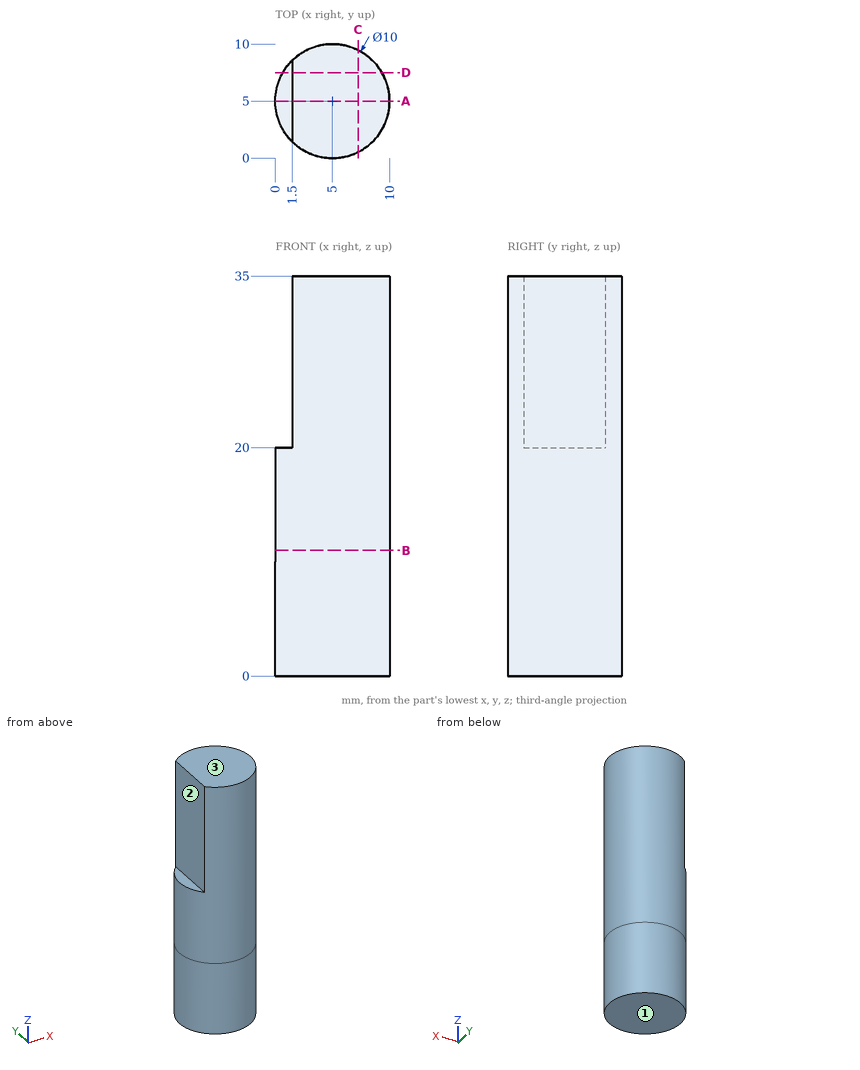
Study the drawing (mm; zero at the part's minimum x, y, z) and answer. Give positions to 0.01 mm unless a question says otherwise; leave off trailing zeros. Write each loop counter-clockwise with the first axis right and the second up, starting at its lowest first coordinate (ties: lowest second). Pieces come first, ordered by that corner, then holes. Notation, with made-up numbers: (51, 46.25) -> (79, 46.25) arc R20 ccw to (79, 57.25) -> close; hole circle Ø6 at (31, 33.25). An arc over 180 degrees is marked (long way). Answer in a Markdown table with one row per item.
1) Determine the mould class of the marked faces 1, 2 and 3 for opening direction Z: released by +Z, released by -Z, zero draft, split by the parting line, or undercut.
Results list:
| item | result |
|---|---|
| face 1 | released by -Z |
| face 2 | zero draft |
| face 3 | released by +Z |
2) Section D-D on y = 7.5 is taken. Give the vertices of the cut face in (x, z), plus the area to 3 significant figures.
Results list:
| item | result |
|---|---|
| outline | (0.67, 0) -> (9.33, 0) -> (9.33, 35) -> (1.5, 35) -> (1.5, 20) -> (0.67, 20) -> close |
| area | 291 mm^2 |
3) Section C-C on x = 7.25 is taken. Give the vertices of the cut face in (y, z).
Results list:
| item | result |
|---|---|
| outline | (0.53, 0) -> (9.47, 0) -> (9.47, 35) -> (0.53, 35) -> close |
4) Each of these flat-tipped pins is pushed along its axis until it touches: pin 1 Ø1.5 at (x, z) = (3, 6.5) entering from -Y; pin 2 Ø0.8 at (x, y) = (1, 4) entering from +Z; pin 3 Ø2 at (y, z) = (6.5, 12) entering from -X; pin 4 Ø1 at (x, y) = (3.5, 7.5) entering from -Z. Where does it stop, or does it pass through?
Results list:
| item | result |
|---|---|
| pin 1 | y = 0.16 |
| pin 2 | z = 20 |
| pin 3 | x = 0.03 |
| pin 4 | z = 0 |
5) Section A-A on y = 5 is taken. Give the vertices of the cut face in (x, z).
Results list:
| item | result |
|---|---|
| outline | (0, 0) -> (10, 0) -> (10, 35) -> (1.5, 35) -> (1.5, 20) -> (0, 20) -> close |
6) Section B-B on z = 11 is taken. Give the vertices of the cut face in (x, y), plus the area to 3 significant figures.
Results list:
| item | result |
|---|---|
| outline | circle Ø10 at (5, 5) |
| area | 78.5 mm^2 |
7) Straight lines are drawn through the part: line 1 (X direction, y = 5.25, z = 31); line 2 (X direction, y = 1.5, z = 31); line 3 (Y direction, x = 2.5, z = 22.5). For each, find the intervals that lie inside material, in ascending order. Write a range as [from, to].
Results list:
| item | result |
|---|---|
| line 1 | [1.5, 9.99] |
| line 2 | [1.5, 8.57] |
| line 3 | [0.67, 9.33] |
